For this review, use the dimensioned drawing (mm, ordinates from the lowest corner) and the shaded views. A direction names the side the tool comes from. Give positions to 0.01 mm unless a question says otherwise; leave off trailing zeros. Order: outer loops, then holes, each group sorted by start corner. A loop starts at its lowest first (then second) coordinate and runs counter-clockwise, first axis right, second up. Notation, with made-up numbers: (-32, 14.5) -> (8, 14.5) arc R24 ccw to (8, 31.5) -> close; hole circle Ø4 at (-29, 55.5). An arc over 180 degrees is marked (long way). Return JSON: item names as keys, results as strings.
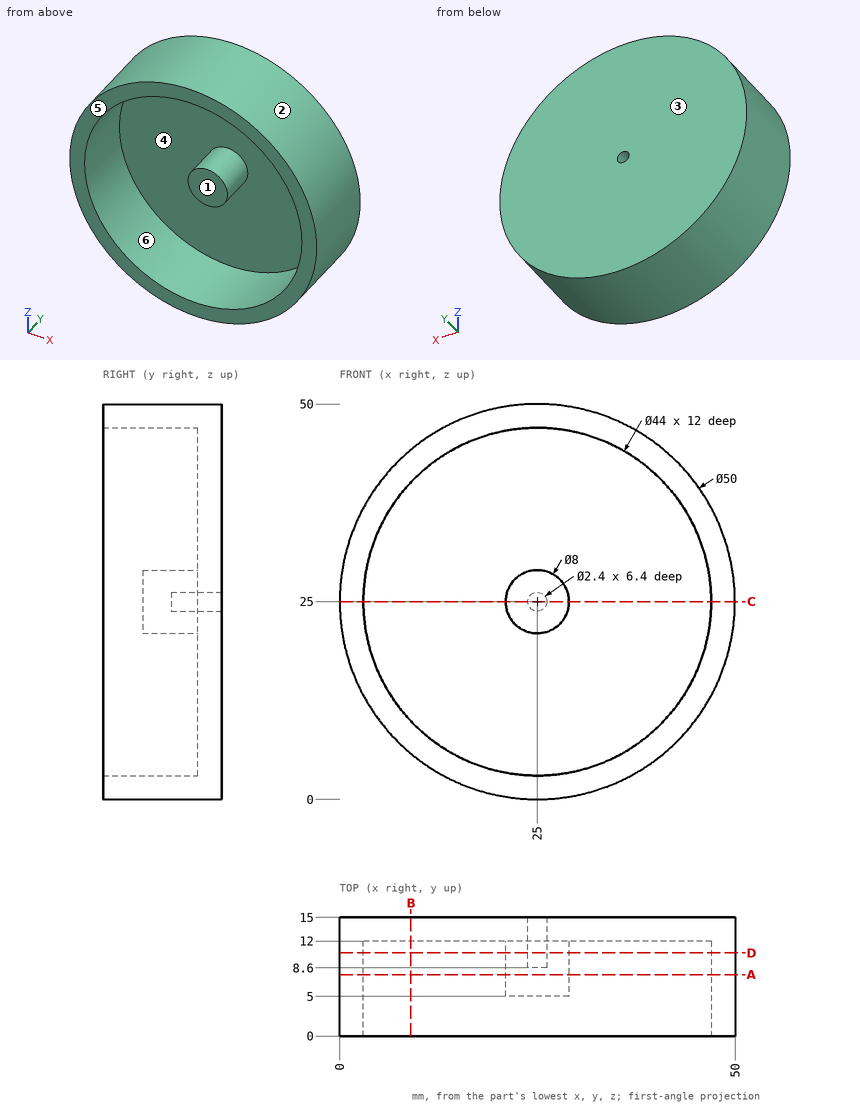
Item 1: Machinability: for the marked faces 5 and 6, which of the approach directions +Z, -Z, +X, -X, +Y, -Y give a long, thin tool a straight path to every point of the face, cutting with its end or side? Answer none if there is none.
Result set:
{"face 5": "+Z, -Z, +X, -X, -Y", "face 6": "-Y"}
Item 2: Wall thickness on L1, parallel to Z at x = 25, y = 11.75; L2, parallel to X at y = 11.5, z = 28; L3, parallel to X at y = 8, z = 23: over which ranges is each line inside the solid? List them lowest first. Write a range as [from, to].
Result set:
{"L1": "z = [0, 3], [21, 23.8], [26.2, 29], [47, 50]", "L2": "x = [0.18, 3.21], [22.35, 27.65], [46.79, 49.82]", "L3": "x = [0.08, 3.09], [21.54, 28.46], [46.91, 49.92]"}
Item 3: Add section C-C (z = 25). Give the boundary of the cut face in (x, y), plus the area to 3 significant figures.
Result set:
{"outline": "(0, 0) -> (3, 0) -> (3, 12) -> (21, 12) -> (21, 5) -> (29, 5) -> (29, 12) -> (47, 12) -> (47, 0) -> (50, 0) -> (50, 15) -> (26.2, 15) -> (26.2, 8.6) -> (23.8, 8.6) -> (23.8, 15) -> (0, 15) -> close", "area": "263 mm^2"}
Item 4: Mouldability with a two-part tool opening along Z and no side actions: class the marked faces 1, 2, 3 and 4 as released by +Z, released by -Z, zero draft, split by the parting line, or undercut.
Result set:
{"face 1": "undercut", "face 2": "split by the parting line", "face 3": "zero draft", "face 4": "undercut"}
Item 5: For pin 1 (2 mm diameter, centred on x = 25, z = 25, fed in from +Y); pin 2 (1 mm diameter, centred on x = 8.5, z = 25, fed in from -Y); pin 3 (9 mm diameter, centred on x = 24.5, z = 23, fed in from -Y), all flat-tipped, find the tip position at first contact; note any pin that passes through.
Result set:
{"pin 1": "stops at y = 8.6", "pin 2": "stops at y = 12", "pin 3": "stops at y = 5"}
Item 6: Add section D-D (y = 10.5). Give the boundary of the cut face in (x, z), plus the area to 3 significant figures.
Result set:
{"outline": "circle Ø50 at (25, 25); circle Ø8 at (25, 25); hole circle Ø44 at (25, 25); hole circle Ø2.4 at (25, 25)", "area": "489 mm^2"}
Item 7: Add section B-B (x = 9). Give the boundary of the cut face in (y, z), plus the area to 3 significant figures.
Result set:
{"outline": "(0, 5.79) -> (15, 5.79) -> (15, 44.21) -> (0, 44.21) -> (0, 40.1) -> (12, 40.1) -> (12, 9.9) -> (0, 9.9) -> close", "area": "214 mm^2"}
Item 8: Add section A-A (y = 7.75). Give the boundary of the cut face in (x, z).
Result set:
{"outline": "circle Ø50 at (25, 25); circle Ø8 at (25, 25); hole circle Ø44 at (25, 25)"}
